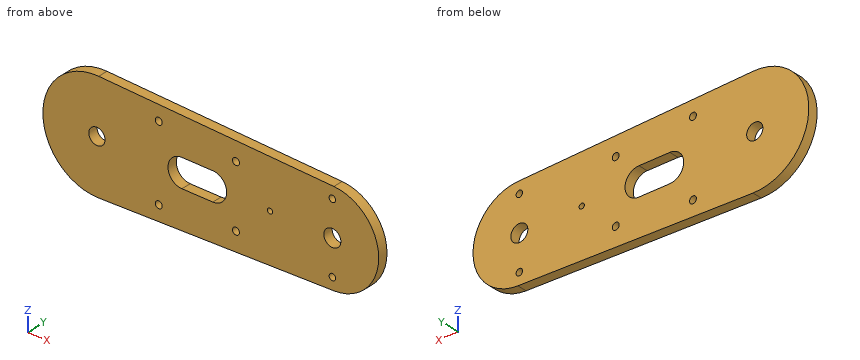
```python
from build123d import *

# Parameters (mm, degrees)
PLACA_START                         = -10.35
PLACA_DEPTH                         = 6.35
PLACA_R1_START                      = -10.35
CROQUIS2_R                          = 35
PLACA_R1_DEPTH                      = 6.35
PLACA_R2_START                      = -10.35
CROQUIS3_R                          = 30
PLACA_R2_DEPTH                      = 6.35
ALIGERADO_START                     = -10.35
ALIGERADO_DEPTH                     = 6.35
BARRENOS_SEPARADORES_M4_START       = -10.35
CROQUIS5_R                          = 2.25
BARRENOS_SEPARADORES_M4_DEPTH       = 6.35
PASO_PERNOS_Y_ROSCA_M5_KFL000_START = -10.35
CROQUIS6_R                          = 5.25
CROQUIS6_R_2                        = 5.5
CROQUIS6_R_3                        = 2.1
PASO_PERNOS_Y_ROSCA_M5_KFL000_DEPTH = 6.35
ROSCA_M3_BASES_CINCHO_START         = -10.35
CROQUIS7_R                          = 1.25
ROSCA_M3_BASES_CINCHO_DEPTH         = 6.35
PASO_M3_BASES_CINCHO_START          = -10.35
CROQUIS8_R                          = 1.7
PASO_M3_BASES_CINCHO_DEPTH          = 6.35


with BuildPart() as part:
    # Croquis1 → Placa (new body)
    with BuildSketch(Plane(origin=(0, 0, 0), x_dir=(1, 0, 0), z_dir=(0, 1, 0)).offset(PLACA_START)):
        Polygon((1.148293963, -206.431158085), (153.384251969, -201.433849787), (153.384251969, -141.466150213), (1.148293963, -136.468841915), align=None)
    extrude(amount=PLACA_DEPTH)

    # Croquis2 → Placa_r1 (add)
    with BuildSketch(Plane(origin=(0, 0, 0), x_dir=(1, 0, 0), z_dir=(0, 1, 0)).offset(PLACA_R1_START)):
        with Locations((0, -171.45)):
            Circle(CROQUIS2_R)
    extrude(amount=PLACA_R1_DEPTH)

    # Croquis3 → Placa_r2 (add)
    with BuildSketch(Plane(origin=(0, 0, 0), x_dir=(1, 0, 0), z_dir=(0, 1, 0)).offset(PLACA_R2_START)):
        with Locations((152.4, -171.45)):
            Circle(CROQUIS3_R)
    extrude(amount=PLACA_R2_DEPTH)

    # Croquis4 → Aligerado (cut)
    with BuildSketch(Plane(origin=(0, 0, 0), x_dir=(1, 0, 0), z_dir=(0, 1, 0)).offset(ALIGERADO_START)):
        with BuildLine():
            Line((55, -162.45), (75, -162.45))
            ThreePointArc((75, -162.45), (84, -171.45), (75, -180.45))
            Line((75, -180.45), (55, -180.45))
            ThreePointArc((55, -180.45), (46, -171.45), (55, -162.45))
        make_face()
    extrude(amount=ALIGERADO_DEPTH, mode=Mode.SUBTRACT)

    # Croquis5 → Barrenos_separadores_M4 (cut)
    with BuildSketch(Plane(origin=(0, 0, 0), x_dir=(1, 0, 0), z_dir=(0, 1, 0)).offset(BARRENOS_SEPARADORES_M4_START)):
        with Locations(Location((40, -195.45, 0), (0, 0, 270))):
            Circle(CROQUIS5_R)
        with Locations(Location((40, -147.45, 0), (0, 0, 270))):
            Circle(CROQUIS5_R)
        with Locations(Location((90, -191.45, 0), (0, 0, 270))):
            Circle(CROQUIS5_R)
        with Locations(Location((90, -151.45, 0), (0, 0, 270))):
            Circle(CROQUIS5_R)
    extrude(amount=BARRENOS_SEPARADORES_M4_DEPTH, mode=Mode.SUBTRACT)

    # Croquis6 → Paso_pernos_y_rosca_M5_KFL000 (cut)
    with BuildSketch(Plane(origin=(0, 0, 0), x_dir=(1, 0, 0), z_dir=(0, 1, 0)).offset(PASO_PERNOS_Y_ROSCA_M5_KFL000_START)):
        with Locations(Location((0, -171.45, 0), (0, 0, 270))):
            Circle(CROQUIS6_R)
        with Locations(Location((152.4, -171.45, 0), (0, 0, 270))):
            Circle(CROQUIS6_R_2)
        with Locations(Location((152.4, -193.95, 0), (0, 0, 270))):
            Circle(CROQUIS6_R_3)
        with Locations(Location((152.4, -148.95, 0), (0, 0, 270))):
            Circle(CROQUIS6_R_3)
    extrude(amount=PASO_PERNOS_Y_ROSCA_M5_KFL000_DEPTH, mode=Mode.SUBTRACT)

    # Croquis7 → Rosca_M3_bases_cincho (cut)
    with BuildSketch(Plane(origin=(0, 0, 0), x_dir=(1, 0, 0), z_dir=(0, 1, 0)).offset(ROSCA_M3_BASES_CINCHO_START)):
        with Locations(Location((112, -171.45, 0), (0, 0, 270))):
            Circle(CROQUIS7_R)
    extrude(amount=ROSCA_M3_BASES_CINCHO_DEPTH, mode=Mode.SUBTRACT)

    # Croquis8 → Paso_M3_bases_cincho (cut)
    with BuildSketch(Plane(origin=(0, 0, 0), x_dir=(1, 0, 0), z_dir=(0, 1, 0)).offset(PASO_M3_BASES_CINCHO_START)):
        with Locations(Location((112, -171.45, 0), (0, 0, 270))):
            Circle(CROQUIS8_R)
    extrude(amount=PASO_M3_BASES_CINCHO_DEPTH, mode=Mode.SUBTRACT)


solid = part.part
```
Can you work these out from the model? Positions are in its coordinate system, mm. Round coordinates to 2 decimals unless told otherwise and drop trailing zeros. Loops run counter-clockwise (first coordinate to the right, second up) from the corner with the lowest first, then second, coordinate; pieces in that order, holes last.
Item 1: Suppose I cut it at A-A, the plane y = -7.5. State how many separate pieces and enclosed holes the cut face has, then the cut area to 3 significant figures.
Item 2: Please list where these lines run through material, in increasing order: L1, parallel to X at y = -5.25, z = 171.45; L2, parallel to X at y = -9.5, z = 170; L3, parallel to X at y = -4.5, z = 168.
Item 3: Suppose I cut it at B-B, the plane x = 90. Write out the boundary of the cut face in (y, z).
Item 4: Will these pins go through, and if not, where does the flat tip stop? pin 1 Ø1 at (x, y) = (39.5, -8.5) entering from -Z; pin 2 Ø1.9 at (x, y) = (67.5, -7.5) entering from -Z; pin 3 Ø2 at (x, y) = (70.5, -5.5) entering from -Z.
Item 5: Suppose I cut it at C-C, the plane z = 187. Write out the boundary of the cut face in (x, y), then the cut area to 3 significant figures.
Reported:
1. separate pieces: 1
1. enclosed holes: 10
1. area: 12,400 mm2
2. L1: x = -35 to -5.25, 5.25 to 46, 84 to 110.3, 113.7 to 146.9, 157.9 to 182.4
2. L2: x = -34.97 to -5.05, 5.05 to 46.12, 83.88 to 111.11, 112.89 to 147.09, 157.71 to 182.36
2. L3: x = -34.83 to -3.96, 3.96 to 46.69, 83.31 to 148.12, 156.68 to 182.2
3. outline: (-10.35, 139.39) - (-4, 139.39) - (-4, 149.2) - (-10.35, 149.2) - close; (-10.35, 153.7) - (-4, 153.7) - (-4, 189.2) - (-10.35, 189.2) - close; (-10.35, 193.7) - (-4, 193.7) - (-4, 203.51) - (-10.35, 203.51) - close
4. pin 1: stops at z = 137.71
4. pin 2: stops at z = 138.62
4. pin 3: stops at z = 138.71
5. outline: (-31.36, -10.35) - (178.06, -10.35) - (178.06, -4) - (-31.36, -4) - close
5. area: 1,330 mm2
